Build history of the part. All positions in model axes, mm. A direction names the side the tool comes from. Round coordinates to 2 decimals unless told otherwise and drop trailing zeros. Write each loop counter-clockwise with the first axis right and the second up, starting at its lowest first coordinate (ties: lowest second). Pieces come first, ordered by that corner, then holes. Notation, with made-up numbers: (65.5, 45) - (89.5, 45) arc R36 cw to (89.5, 81) - close; hole circle Ø5 at (58.5, -4). An arc over 180 degrees is marked (long way). Write each question's results on one line, items separated by ' | '.
from build123d import *

# Parameters (mm, degrees)
BOSS_EXTRU_1_DEPTH      = 5
ESQUISSE3_R             = 2.5
ENL_V_MAT_EXTRU_1_DEPTH = 5
ESQUISSE4_R             = 2.5
ENL_V_MAT_EXTRU_2_DEPTH = 5


with BuildPart() as part:
    # Esquisse2 → Boss.-Extru.1 (new body)
    with BuildSketch(Plane(origin=(0, 0, 0), x_dir=(1, 0, 0), z_dir=(0, 1, 0))):
        with BuildLine():
            ThreePointArc((-4.698463104, -1.710100717), (-4.095760221, 2.867882182), (0, 5))
            Line((0, 5), (3.501037691, 5))
            Line((3.501037691, 5), (-10.692443346, 43.996268652))
            ThreePointArc((-10.692443346, 43.996268652), (-17.101007166, 46.984631039), (-20.089369554, 40.576067219))
            Line((-20.089369554, 40.576067219), (-4.698463104, -1.710100717))
        make_face()
        with BuildLine():
            Line((55, 5), (3.501037691, 5))
            Line((3.501037691, 5), (4.698463104, 1.710100717))
            ThreePointArc((4.698463104, 1.710100717), (4.095760221, -2.867882182), (0, -5))
            Line((0, -5), (55, -5))
            ThreePointArc((55, -5), (60, 0), (55, 5))
        make_face()
        with BuildLine():
            Line((3.501037691, 5), (0, 5))
            ThreePointArc((0, 5), (-4.095760221, 2.867882182), (-4.698463104, -1.710100717))
            ThreePointArc((-4.698463104, -1.710100717), (-2.867882182, -4.095760221), (0, -5))
            ThreePointArc((0, -5), (4.095760221, -2.867882182), (4.698463104, 1.710100717))
            Line((4.698463104, 1.710100717), (3.501037691, 5))
        make_face()
    extrude(amount=BOSS_EXTRU_1_DEPTH)

    # Esquisse3 → Enlèv. mat.-Extru.1 (cut)
    with BuildSketch(Plane(origin=(0, 5, 0), x_dir=(1, 0, 0), z_dir=(0, 1, 0))):
        with Locations(Location((-15.39090645, 42.286167935, 0), (0, 0, 270))):
            Circle(ESQUISSE3_R)
        with Locations(Location((55, 0, 0), (0, 0, 270))):
            Circle(ESQUISSE3_R)
    extrude(amount=-ENL_V_MAT_EXTRU_1_DEPTH, mode=Mode.SUBTRACT)

    # Esquisse4 → Enlèv. mat.-Extru.2 (cut)
    with BuildSketch(Plane(origin=(0, 5, 0), x_dir=(1, 0, 0), z_dir=(0, 1, 0))):
        with Locations(Location((0, 0, 0), (0, 0, 270))):
            Circle(ESQUISSE4_R)
    extrude(amount=-ENL_V_MAT_EXTRU_2_DEPTH, mode=Mode.SUBTRACT)


solid = part.part
(1) Slice it at D-D, the plane x = 28. Write the cut outline in (y, z).
Worked answers:
outline: (0, -5) - (5, -5) - (5, 5) - (0, 5) - close
(2) Slice it at B-B, the plane y = 3.1. Write the cut outline in (x, z), and give its area (3 significant figures).
Worked answers:
outline: (-20.09, -40.58) arc R5 ccw to (-10.69, -44) - (3.5, -5) - (55, -5) arc R5 ccw to (55, 5) - (0, 5) arc R5 ccw to (-4.7, 1.71) - close; hole circle Ø5 at (-15.39, -42.29); hole circle Ø5 at (0, 0); hole circle Ø5 at (55, 0) | area: 1,020 mm2
(3) Drill centre lines: probe 1 along X at (y, z) = (1.5, 0); probe 2 along Z at (x, y) = (16.5, 1.7); probe 3 along X at (y, z) = (4.1, -43). Where is each one in solid material? Low to high. Write a range as [from, to].
Worked answers:
probe 1: x = [-5.32, -2.5], [2.5, 52.5], [57.5, 60] | probe 2: z = [-5, 5] | probe 3: x = [-20.34, -17.79], [-12.99, -10.33]
(4) Slice it at A-A, the plane z = 0. Write the cut outline in (x, y), and give its area (3 significant figures).
Worked answers:
outline: (-5.32, 0) - (-2.5, 0) - (-2.5, 5) - (-5.32, 5) - close; (2.5, 0) - (52.5, 0) - (52.5, 5) - (2.5, 5) - close; (57.5, 0) - (60, 0) - (60, 5) - (57.5, 5) - close | area: 277 mm2
(5) Slice it at C-C, the plane x = 1.5. Write the cut outline in (y, z).
Worked answers:
outline: (0, -10.5) - (5, -10.5) - (5, -2) - (0, -2) - close; (0, 2) - (5, 2) - (5, 5) - (0, 5) - close
(6) Two-plate mould, pull along X, no slides. Class faces 3 (the cylindrical face through (-16.348, 2.535, -39.977)), 4 (the cylindrical face through (60, 2, 0)), 5 (the cylindrical face through (-3, 2, 4)): released by +X, released by -X, zero draft, split by the parting line, or undercut.
Worked answers:
face 3: undercut | face 4: released by +X | face 5: released by -X
(7) Tool access for faces 1 (the flat face through (30, 2, -5)), 2 (the cylindrical face through (52.56, 2.54, -0.54)): list every direction of +Z, -Z, +X, -X, +Y, -Y with a clear straight run to the whole face (end or side of a thin tool).
Worked answers:
face 1: -Z, +X, +Y, -Y | face 2: +Y, -Y
(8) Flat gauge pins, fed straight in: pin 1 Ø3 at (x, y) = (11, 3.5) entering from -Z; pin 2 Ø1 at (y, z) = (4, -18.5) entering from +X; pin 3 Ø2 at (y, z) = (0.5, -37) entering from +X. Where does each tip first touch, or does it go through?
Worked answers:
pin 1: stops at z = -5 | pin 2: stops at x = -1.23 | pin 3: stops at x = -7.78
